Check sheet for the modelled part. Datum: model origin and axes. Units: mm. A direction names the side the tool comes from. Give positions to 0.01 mm unless a question says otherwise; leave off trailing zeros. Order: outer loops, then holes, each group sorted by start corner. A loop starts at its lowest first (then second) coordinate and runs counter-clockwise, first axis right, second up.
Item 1: Sectioned sample at A-A on x = 0. Record the boundary of the cut face in (y, z), and give its area (3 significant figures).
Item 2: Sectioned sample at C-C on y = 26.5. Record the boundary of the cut face in (x, z).
Item 3: Release check for a two-part mould opening along X. For faces 1 (the flat face through (-6.09, 63.99, 3.45)), 2 (the conical face through (48.154, 0.486, -15.164)), 3 (the cylindrical face through (19.129, 2.535, 29.406)) record: released by +X, released by -X, zero draft, split by the parting line, or undercut.
Item 4: Material ranges on line 1 along Z through (x, y) = (-18, 1.45); line 2 along Z through (x, y) = (18, 2.9); line 3 along Y through (x, z) = (6, -42.5), recorded low to high.
Item 5: Sectioned sample at B-B on y = 61.5. Record the boundary of the cut face in (x, z).
Item 6: Gauge pin test, flat ends, axial feed: P1, Ø4, axis at x = 1.5, y = 65, coming from the +Z side; P2, Ø4, axis at x = -30, z = -26, coming from the +Y side; P3, Ø1, axis at y = 24, z = 2, coming from the -X side; P4, Ø5.5, axis at x = -18, z = -31.18, coming from the -Y side. Record the tip position at first contact, or that the pin passes through.
Item 7: Access from +Z, -Z, +X, -X, +Y, -Y to the whole of each face (thin tool, end or side, straight path). Record for faces 4 (the flat face through (6.034, 63.99, 3.549)), 5 (the flat face through (0, 64, -7)), 6 (the cylindrical face through (-17.031, 2.535, -29.314)), 7 (the flat face through (0, 64, 7)).
from build123d import *

# Parameters (mm, degrees)
SKETCH1_R                       = 60
BOSS_EXTRUDE1_DEPTH             = 49.2
BOSS_EXTRUDE3_DEPTH             = 30
FILLET1_R                       = 5
TAP_DRILL_FOR_M5X0_8_TAP1_D     = 4.2
TAP_DRILL_FOR_M5X0_8_TAP1_DEPTH = 5
TAP_DRILL_FOR_M5X0_8_TAP1_TIP   = 1.2618073
CHAMFER1_SIZE                   = 10


with BuildPart() as part:
    # Sketch1 → Boss-Extrude1 (new body)
    with BuildSketch(Plane(origin=(0, 0, 0), x_dir=(1, 0, 0), z_dir=(0, 1, 0))):
        Circle(SKETCH1_R)
    extrude(amount=BOSS_EXTRUDE1_DEPTH)

    # Sketch2 → Boss-Extrude3 (add)
    with BuildSketch(Plane(origin=(0, 49.2, 0), x_dir=(1, 0, 0), z_dir=(0, 1, 0))):
        Polygon((-4.041451884, 7), (-8.082903769, 0), (-4.041451884, -7), (4.041451884, -7), (8.082903769, 0), (4.041451884, 7), align=None)
    extrude(amount=BOSS_EXTRUDE3_DEPTH)

    # Fillet1
    fillet1_edges = [part.edges().sort_by_distance(p)[0] for p in [
        (-60, 49.2, 0),
    ]]
    fillet(fillet1_edges, radius=FILLET1_R)

    # Tap Drill for M5x0.8 Tap1
    with Locations(Plane(origin=(0, 0, 0), x_dir=(-1, 0, 0), z_dir=(0, -1, 0))):
        with Locations((-18, 31.176914536), (18, 31.176914536), (18, -31.176914536), (-18, -31.176914536)):
            Hole(TAP_DRILL_FOR_M5X0_8_TAP1_D / 2, depth=TAP_DRILL_FOR_M5X0_8_TAP1_DEPTH)
            with Locations((0, 0, -(TAP_DRILL_FOR_M5X0_8_TAP1_DEPTH + TAP_DRILL_FOR_M5X0_8_TAP1_TIP / 2))):  # 118° drill point
                Cone(0, TAP_DRILL_FOR_M5X0_8_TAP1_D / 2, TAP_DRILL_FOR_M5X0_8_TAP1_TIP, mode=Mode.SUBTRACT)

    # Chamfer1
    chamfer1_edges = [part.edges().sort_by_distance(p)[0] for p in [
        (-60, 0, 0),
    ]]
    chamfer(chamfer1_edges, length=CHAMFER1_SIZE)


solid = part.part
Report:
1. outline: (0, -50) - (10, -60) - (44.2, -60) arc R5 ccw to (49.2, -55) - (49.2, -7) - (79.2, -7) - (79.2, 7) - (49.2, 7) - (49.2, 55) arc R5 ccw to (44.2, 60) - (10, 60) - (0, 50) - close
1. area: 6,210 mm2
2. outline: circle Ø120 at (0, 0)
3. face 1: released by -X
3. face 2: split by the parting line
3. face 3: undercut
4. line 1: z = -48.2 to -33.28, -29.08 to 29.08, 33.28 to 48.2
4. line 2: z = -49.74 to -33.28, -29.08 to 29.08, 33.28 to 49.74
4. line 3: y = 0 to 49.2
5. outline: (-8.08, 0) - (-4.04, -7) - (4.04, -7) - (8.08, 0) - (4.04, 7) - (-4.04, 7) - close
6. P1: stops at z = 7
6. P2: stops at y = 49.2
6. P3: stops at x = -59.98
6. P4: stops at y = 0
7. face 4: +Z, +X, +Y
7. face 5: -Z, +X, -X, +Y
7. face 6: -Y
7. face 7: +Z, +X, -X, +Y
